Build history of the part. All positions in model axes, mm. Face numbers are marked on the shaded views. A direction names the side the tool comes from. Round coordinates to 2 decimals unless told otherwise and drop trailing zeros. Write each loop counter-clockwise with the first axis right and the second up, starting at its lowest first coordinate (ties: lowest second). Pieces come first, ordered by that corner, then holes. Notation, with made-up numbers: (80.25, 10.5) - (106.25, 10.5) arc R7 ccw to (106.25, 23.5) - close; hole circle Ø6 at (39.5, 5.5). An arc over 180 degrees is marked (long way). One line per question, with ' | ' between items.
from build123d import *

# Parameters (mm, degrees)
SKETCH1_W           = 40.9
SKETCH1_H           = 22.2
SKETCH1_R           = 2.25
SKETCH1_R_2         = 2.75
BOSS_EXTRUDE4_DEPTH = 20
SKETCH4_W           = 70.9
SKETCH4_H           = 15.47309833
CUT_EXTRUDE1_DEPTH  = 15


with BuildPart() as part:
    # Sketch1 → Boss-Extrude4 (new body)
    with BuildSketch(Plane.XY):
        Polygon((-35.45, 22.62690167), (-35.45, -22.62690167), (35.45, -26.57309833), (35.45, 26.57309833), align=None)
        Rectangle(SKETCH1_W, SKETCH1_H, mode=Mode.SUBTRACT)
        with Locations((-20.95, 17.6)):
            Circle(SKETCH1_R, mode=Mode.SUBTRACT)
        with Locations((20.95, 19.932096475)):
            Circle(SKETCH1_R, mode=Mode.SUBTRACT)
        with Locations((-24.2, 4.86)):
            Circle(SKETCH1_R_2, mode=Mode.SUBTRACT)
        with Locations((-24.2, -4.86)):
            Circle(SKETCH1_R_2, mode=Mode.SUBTRACT)
        with Locations((24.2, 4.86)):
            Circle(SKETCH1_R_2, mode=Mode.SUBTRACT)
        with Locations((24.2, -4.86)):
            Circle(SKETCH1_R_2, mode=Mode.SUBTRACT)
        with Locations((20.95, -19.932096475)):
            Circle(SKETCH1_R, mode=Mode.SUBTRACT)
        with Locations((-20.95, -17.6)):
            Circle(SKETCH1_R, mode=Mode.SUBTRACT)
    extrude(amount=BOSS_EXTRUDE4_DEPTH)

    # Sketch4 → Cut-Extrude1 (cut)
    with BuildSketch(Plane.XY.offset(20)):
        with Locations((0, 18.836549165)):
            Rectangle(SKETCH4_W, SKETCH4_H)
        with Locations((0, -18.836549165)):
            Rectangle(SKETCH4_W, SKETCH4_H)
    extrude(amount=-CUT_EXTRUDE1_DEPTH, mode=Mode.SUBTRACT)


solid = part.part
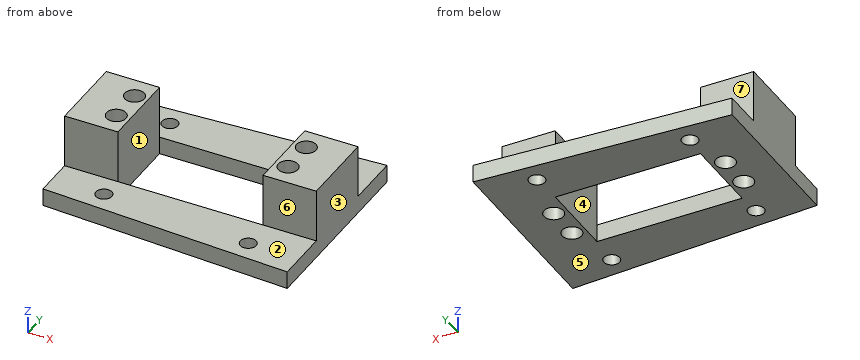
Q1. Saw through at B-B, the plane y = -4.86. List the corners of the cut face in (x, z), then the cut area to 3 significant figures.
Found:
outline: (-35.45, 0) - (-26.95, 0) - (-26.95, 20) - (-35.45, 20) - close; (-21.45, 0) - (-20.45, 0) - (-20.45, 20) - (-21.45, 20) - close; (20.45, 0) - (21.45, 0) - (21.45, 20) - (20.45, 20) - close; (26.95, 0) - (35.45, 0) - (35.45, 20) - (26.95, 20) - close | area: 380 mm^2
Q2. Which spindle directions (+Z, -Z, +X, -X, +Y, -Y) get a long thin tool onto all of the face, cutting with end or side? Do the marked faces 5, 6 and 7. Say none if no direction does.
Found:
face 5: -Z, +X, -X, +Y, -Y | face 6: +Z, +X, -X, -Y | face 7: +Z, +X, -X, +Y
Q3. Pull direction X, two halves, no side cores. Call the marked faces 1, 2, 3 and 4: +X half, -X half, draft (parallel to the pull), parting line (faces both ways), or undercut.
Found:
face 1: undercut | face 2: draft | face 3: +X half | face 4: undercut
Q4. Saw through at D-D, the plane y = -19. List the corners of the cut face in (x, z), then the cut area to 3 significant figures.
Found:
outline: (-35.45, 0) - (-22.71, 0) - (-22.71, 5) - (-35.45, 5) - close; (-19.19, 0) - (18.9, 0) - (18.9, 5) - (-19.19, 5) - close; (23, 0) - (35.45, 0) - (35.45, 5) - (23, 5) - close | area: 316 mm^2
Q5. Saw through at C-C, the plane x = 8.5. List the corners of the cut face in (y, z), then the cut area to 3 significant figures.
Found:
outline: (-25.07, 0) - (-11.1, 0) - (-11.1, 5) - (-25.07, 5) - close; (11.1, 0) - (25.07, 0) - (25.07, 5) - (11.1, 5) - close | area: 140 mm^2
Q6. Drill centre lines: L1, parallel to Y at x = -24.2, z = 13.25; L2, parallel to X at y = 10, z = 5.25; L3, parallel to Y at x = -20.95, z = 2.8. Where is each one in solid material? Low to high. Write a range as from..to.
Found:
L1: -11.1..-7.61, -2.11..2.11, 7.61..11.1 | L2: -35.45..-20.45, 20.45..35.45 | L3: -23.43..-19.85, -15.35..15.35, 19.85..23.43
Q7. Drop flat-ended pins along their axis: pin 1 (12 mm diameter, centred on x = -29.5, z = 14, fed in from +Y); pin 2 (12.5 mm diameter, centred on x = -10.5, y = 19, fed in from +Z); pin 3 (10 mm diameter, centred on x = -2, z = 11.5, fed in from -Y); pin 4 (2.5 mm diameter, centred on x = -9.5, z = 2.5, fed in from +Y). Give the stop position or say it passes through.
Found:
pin 1: y = 11.1 | pin 2: z = 5 | pin 3: through | pin 4: y = 24.14
Q8. Saw through at A-A, the plane z = 7.25. List the corners of the cut face in (x, y), then the cut area to 3 significant figures.
Found:
outline: (-35.45, -11.1) - (-20.45, -11.1) - (-20.45, 11.1) - (-35.45, 11.1) - close; (20.45, -11.1) - (35.45, -11.1) - (35.45, 11.1) - (20.45, 11.1) - close; hole circle Ø5.5 at (-24.2, -4.86); hole circle Ø5.5 at (-24.2, 4.86); hole circle Ø5.5 at (24.2, -4.86); hole circle Ø5.5 at (24.2, 4.86) | area: 571 mm^2
